```python
from build123d import *

# Parameters (mm, degrees)
BOSS_EXTRUDE1_DEPTH = 6.45
SKETCH2_W           = 25
SKETCH2_H           = 6
BOSS_EXTRUDE2_DEPTH = 2.6
SKETCH3_R           = 3.5
CUT_EXTRUDE1_DEPTH  = 7.45
SKETCH4_R           = 1.4
CUT_EXTRUDE2_DEPTH  = 10.05


with BuildPart() as part:
    # Sketch1 → Boss-Extrude1 (new body)
    with BuildSketch(Plane(origin=(0, 0, 0), x_dir=(1, 0, 0), z_dir=(0, 1, 0))):
        Polygon((5.5, 6), (5.5, 22.5), (-7.5, 22.5), (-7.5, 6), (-17.5, 6), (-17.5, -6), (-7.5, -6), (-7.5, -21.5), (5.5, -21.5), (5.5, -6), (17.5, -6), (17.5, 6), align=None)
    extrude(amount=BOSS_EXTRUDE1_DEPTH)

    # Sketch2 → Boss-Extrude2 (add)
    with BuildSketch(Plane(origin=(0, 6.45, 0), x_dir=(1, 0, 0), z_dir=(0, 1, 0))):
        with Locations((-5, -3)):
            Rectangle(SKETCH2_W, SKETCH2_H)
    extrude(amount=BOSS_EXTRUDE2_DEPTH)

    # Sketch3 → Cut-Extrude1 (cut, through all)
    with BuildSketch(Plane(origin=(0, 6.45, 0), x_dir=(1, 0, 0), z_dir=(0, 1, 0))):
        with Locations((-1, 15)):
            Circle(SKETCH3_R)
        with Locations((-1, -15)):
            Circle(SKETCH3_R)
    extrude(amount=-CUT_EXTRUDE1_DEPTH, mode=Mode.SUBTRACT)

    # Sketch4 → Cut-Extrude2 (cut, through all)
    with BuildSketch(Plane(origin=(0, 9.05, 0), x_dir=(1, 0, 0), z_dir=(0, 1, 0))):
        with Locations((-14.5, -3)):
            Circle(SKETCH4_R)
        with Locations((4.5, -3)):
            Circle(SKETCH4_R)
    extrude(amount=-CUT_EXTRUDE2_DEPTH, mode=Mode.SUBTRACT)


solid = part.part
```
The model under review builds one solid part; all positions refer to its coordinate system, in mm. A direction names the side the tool comes from. Give positions to 0.01 mm unless a question says otherwise; leave off trailing zeros. Write each loop counter-clockwise with the first axis right and the second up, starting at its lowest first coordinate (ties: lowest second). Pieces come first, ordered by that corner, then holes. Notation, with made-up numbers: (71, 46) - (119, 46) arc R19 cw to (119, 50) - close; hole circle Ø1 at (59.5, -25). An arc over 180 degrees is marked (long way). Answer in a Markdown table with one row per item. Add a question column.
1. We need section D-D on y = 1. Write out the cut boundary in (x, z), then the cut area to 3 significant figures.
2. We need section A-A on z = 15. Write out the cut boundary in (x, y).
3. Wall thickness on line 1 along Z through (x, y) = (-1, 3.5); line 2 along X through (y, z) = (2, 15); line 3 along X through (y, z) = (5.5, 3): over which ranges is each line inside the solid? List them lowest first. Write a range as [from, to].
4. Insertion check: P1, Ø12, axis at x = 4, z = 14.5, coming from the +Y side; P2, Ø3, axis at y = 4.5, z = -11.5, coming from the -X side; P3, Ø2, axis at y = 7.5, z = 2.5, coming from the +X side. Each pin has a flat end and moves straight along its axis. Give the tip position at first contact, or say it passes through.
5. We need section B-B on x = -14.5. Write out the cut boundary in (y, z), then the cut area to 3 significant figures.
6. We need section C-C on x = -1. Write out the cut boundary in (y, z), then the cut area to 3 significant figures.
7. Tool access review of faces 5 (the flat face through (7.5, 8, 3)), 6 (the flat face through (-5, 8, 0)), 7 (the flat face through (-7.5, 3, -14)): name each direction out of +Z, -Z, +X, -X, +Y, -Y from which nothing blocks a thin tool from reaching the whole face with its end or side.
8. Draft analysis for pull direction X (two halves, no side actions). For faces 1 (the cylindrical face through (4.197, 4.588, 4.367)), 2 (the flat face through (12, 3, -6)), 3 (the cylindrical face through (-1.759, 3.27, 18.417)), 4 (the flat face through (5.5, 3, 14)), state which applies: +X half, -X half, draft (parallel to the pull), parting line (faces both ways), or undercut.
Ans:
| question | item | result |
|---|---|---|
| 1 | outline | (-17.5, -6) - (-7.5, -6) - (-7.5, -22.5) - (5.5, -22.5) - (5.5, -6) - (17.5, -6) - (17.5, 6) - (5.5, 6) - (5.5, 21.5) - (-7.5, 21.5) - (-7.5, 6) - (-17.5, 6) - close; hole circle Ø2.8 at (-14.5, 3); hole circle Ø7 at (-1, -15); hole circle Ø7 at (-1, 15); hole circle Ø2.8 at (4.5, 3) |
| 1 | area | 747 mm^2 |
| 2 | outline | (-7.5, 0) - (-4.5, 0) - (-4.5, 6.45) - (-7.5, 6.45) - close; (2.5, 0) - (5.5, 0) - (5.5, 6.45) - (2.5, 6.45) - close |
| 3 | line 1 | z = [-22.5, -18.5], [-11.5, 11.5], [18.5, 21.5] |
| 3 | line 2 | x = [-7.5, -4.5], [2.5, 5.5] |
| 3 | line 3 | x = [-17.5, -15.9], [-13.1, 3.1], [5.9, 17.5] |
| 4 | P1 | stops at y = 6.45 |
| 4 | P2 | stops at x = -7.5 |
| 4 | P3 | stops at x = 7.5 |
| 5 | outline | (0, -6) - (6.45, -6) - (6.45, 0) - (9.05, 0) - (9.05, 1.6) - (0, 1.6) - close; (0, 4.4) - (9.05, 4.4) - (9.05, 6) - (0, 6) - close |
| 5 | area | 67.7 mm^2 |
| 6 | outline | (0, -22.5) - (6.45, -22.5) - (6.45, -18.5) - (0, -18.5) - close; (0, -11.5) - (6.45, -11.5) - (6.45, 0) - (9.05, 0) - (9.05, 6) - (6.45, 6) - (6.45, 11.5) - (0, 11.5) - close; (0, 18.5) - (6.45, 18.5) - (6.45, 21.5) - (0, 21.5) - close |
| 6 | area | 209 mm^2 |
| 7 | face 5 | +Z, -Z, +X, +Y |
| 7 | face 6 | -Z, +X, -X, +Y |
| 7 | face 7 | -Z, -X, +Y, -Y |
| 8 | face 1 | undercut |
| 8 | face 2 | draft |
| 8 | face 3 | undercut |
| 8 | face 4 | +X half |
